Answer from the drawing. Dimensions are ordinates in mm from the lowest x, y and z of the part. A direction names the side the tool comes from. Round coordinates to 2 decimals unless told otherwise and drop trailing zeros. Order: outer loops, then holes, each group sorted by start corner. A loop starts at its lowest first (then second) coordinate and runs counter-clockwise, first axis right, second up. Notation, with made-up numbers: (48, -15.75) -> (68, -15.75) arc R4 cw to (68, -9.75) -> close; hole circle Ø8 at (-27.5, 26). An arc over 180 degrees is marked (long way). Use a Markdown table: item, result. Add a question column.
Item 1: Flat-ended cylindrical pins translate along their axes: P1, Ø5, axis at x = 90, z = 13, coming from the -Y side; P2, Ø3, axis at x = 17, z = 26, coming from the +Y side. Find the tip coordinate at first contact, or state that the pin passes through.
Item 2: A cutting plane is placed at D-D, the plane y = 35. Determine the outline of the cut face in (x, z).
Item 3: A tool of negligible diameter and unlimited length cuts with its end or side. For the marked faces 1 and 2, from which of +Z, -Z, +X, -X, +Y, -Y can it reach the whole face along a straight path? Write none if from no direction.
Item 4: A cutting plane is placed at B-B, the plane x = 10. Determine the outline of the cut face in (y, z).
Item 5: A cutting plane is placed at A-A, the plane z = 13. Determine the outline of the cut face in (x, y), plus the area to 3 significant figures.
Item 6: A cutting plane is placed at C-C, the plane z = 53. Determine the outline of the cut face in (x, y).
Item 7: Find the intervals of material crossed by L1, parallel to X at y = 3, z = 93; L2, parallel to Y at x = 88, z = 53, in increasing order. Write a range as [from, to].
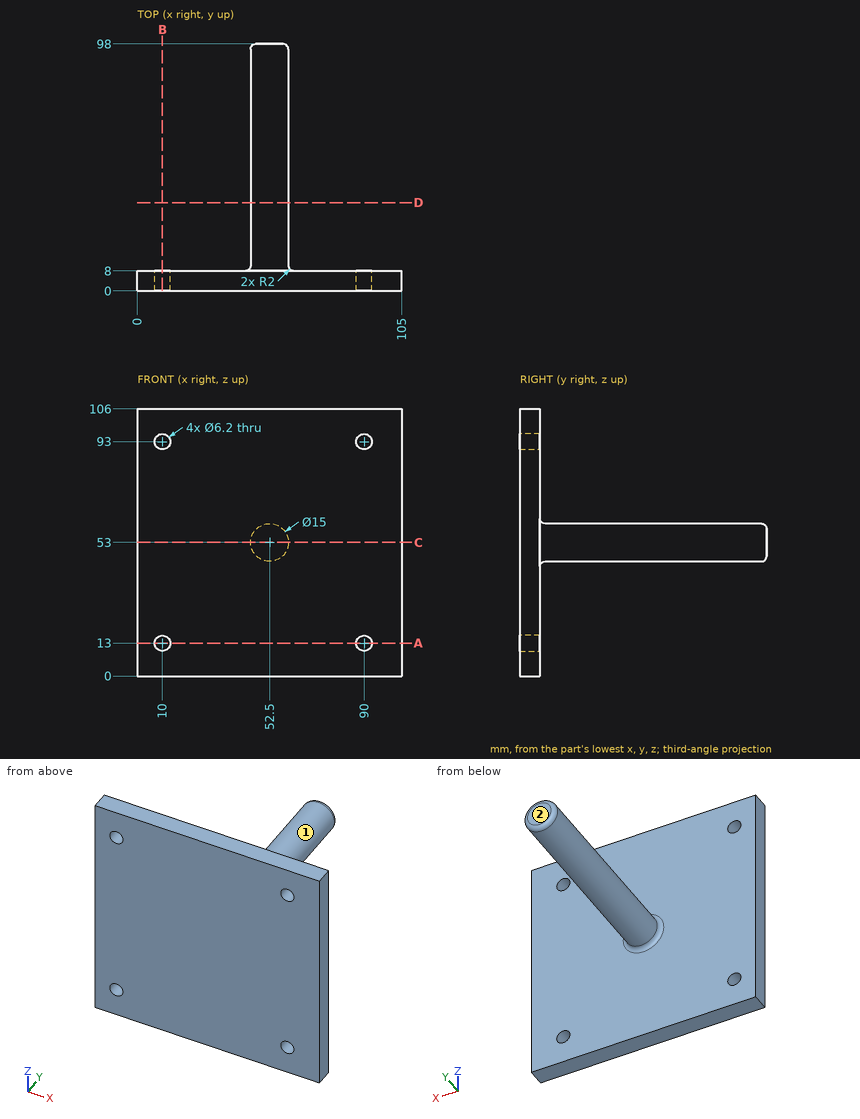
Reported:
| question | item | result |
|---|---|---|
| 1 | P1 | through |
| 1 | P2 | y = 8 |
| 2 | outline | circle Ø15 at (52.5, 53) |
| 3 | face 1 | +Y |
| 3 | face 2 | +Z, -Z, +X, -X, +Y |
| 4 | outline | (0, 0) -> (8, 0) -> (8, 9.9) -> (0, 9.9) -> close; (0, 16.1) -> (8, 16.1) -> (8, 89.9) -> (0, 89.9) -> close; (0, 96.1) -> (8, 96.1) -> (8, 106) -> (0, 106) -> close |
| 5 | outline | (0, 0) -> (6.9, 0) -> (6.9, 8) -> (0, 8) -> close; (13.1, 0) -> (86.9, 0) -> (86.9, 8) -> (13.1, 8) -> close; (93.1, 0) -> (105, 0) -> (105, 8) -> (93.1, 8) -> close |
| 5 | area | 741 mm² |
| 6 | outline | (0, 0) -> (105, 0) -> (105, 8) -> (62, 8) arc R2 cw to (60, 10) -> (60, 96) arc R2 ccw to (58, 98) -> (47, 98) arc R2 ccw to (45, 96) -> (45, 10) arc R2 cw to (43, 8) -> (0, 8) -> close |
| 7 | L1 | [0, 6.9], [13.1, 86.9], [93.1, 105] |
| 7 | L2 | [0, 8] |
